Geometry: final body of the model. Coordinates: model frame, mm. A direction names the side the tool comes from. Give positions to 0.01 mm unless a question says otherwise; leave off trailing zeros. Write each loop counter-clockwise with the first axis right and the second up, starting at its lowest first coordinate (ties: lowest second). Pieces come first, ordered by that corner, then holes. Notation, with made-up numbers: (51, -19.75) -> (63, -19.75) arc R19 cw to (63, 7.25) -> close; hole circle Ø1 at (68, 58). An arc over 180 degrees is marked (long way). Answer as a JSON object with one key per item and string values. Group by question number.
(1) Material intervals for probe 1 along Z at (x, y) = (-48, -4) (3 decimals); probe 2 along X at (y, z) = (-2.4, -96.5); probe 3 along X at (y, z) = (-4.3, -36), sorted ascending.
(2) Section query A-A on x = -40.5. Output: boundary loops of the cut face in (y, z) (3 decimals), plus the area to 3 significant figures.
(3) Section query C-C on y = -1.8. State how many separate pieces and enclosed holes the cut face has, plus the area to 3 significant figures.
(4) Contact query for flat-ended pins moving along their axis: pin 1 Ø0.9 at (y, z) = (-3, 121) entering from +X; pin 2 Ø0.9 at (y, z) = (-2.5, -120.5) entering from -X; pin 3 Ø3 at (y, z) = (-3.5, 120.5) entering from -X; pin 4 Ø6 at (x, z) = (71.5, -25) entering from +Y. Output: stop coordinate, or through.
(5) Section query D-D on x = -102.5. Output: boundary loops of the cut face in (y, z), plus the area to 3 significant figures.
(6) Set-up query: faces 1 (the face through (108.388, -2.504, -63.727)), 2 (the face through (-125.48, -2.58, 27.77)). Return all of +Z, -Z, +X, -X, +Y, -Y with unobstructed straight access to the full face (end or side cutting, diameter ignored); none if empty.
(7) Section query B-B on z = 88. Output: boundary loops of the cut face in (x, y), plus the area to 3 significant figures.
(8) Draft query along X for faces 3 (the face through (125.21, -2.58, 28.24)), 4 (the face through (109.383, -2.504, 62.003)), 5 (the face through (-108.388, -2.504, 63.727)). Return one class per face: +X half, -X half, draft (parallel to the pull), parting line (faces both ways), or undercut.
from build123d import *

# Parameters (mm, degrees)
F1_DEPTH        = 5.08
F2_W            = 38.7485525078
F2_H            = 2.9464
F3_DEPTH        = 5.08
F3_COPIES_COUNT = 6


# Not quite as in the source:
# - a pattern or mirror of a feature is missing from the dataset's text; its kind, count and spacing are read off the source's solid


with BuildPart() as f1:
    # F0 (on Front) → F1 (new body)
    with BuildSketch(Plane.XZ):
        with BuildLine():
            Line((71.1237796615, 125.73), (-71.1237796615, 125.73))
            ThreePointArc((-71.1237796615, 125.73), (-72.3937796615, 125.3897045256), (-73.3234841871, 124.46))
            Line((-73.3234841871, 124.46), (-144.4472638486, 1.27))
            ThreePointArc((-144.4472638486, 1.27), (-144.7875593229, 0), (-144.4472638486, -1.27))
            Line((-144.4472638486, -1.27), (-73.3234841871, -124.46))
            ThreePointArc((-73.3234841871, -124.46), (-72.3937796615, -125.3897045256), (-71.1237796615, -125.73))
            Line((-71.1237796615, -125.73), (71.1237796615, -125.73))
            ThreePointArc((71.1237796615, -125.73), (72.3937796615, -125.3897045256), (73.3234841871, -124.46))
            Line((73.3234841871, -124.46), (144.4472638486, -1.27))
            ThreePointArc((144.4472638486, -1.27), (144.7875593229, 0), (144.4472638486, 1.27))
            Line((144.4472638486, 1.27), (73.3234841871, 124.46))
            ThreePointArc((73.3234841871, 124.46), (72.3937796615, 125.3897045256), (71.1237796615, 125.73))
        make_face()
    extrude(amount=F1_DEPTH)

    # F2 (on face) → F3 (cut, through all)
    with BuildSketch(Plane.XZ.offset(5.08)):
        with Locations((-38.4242762539, 121.0818)):
            Rectangle(F2_W, F2_H)
        with Locations((38.4242762539, 121.0818)):
            Rectangle(F2_W, F2_H)
    f3 = extrude(amount=-F3_DEPTH, mode=Mode.SUBTRACT)

    # F3_copies: F3 ×6 about axis
    f3_copies_axis = Axis((0, 0, 0), (0, 1, 0))
    for i in range(1, F3_COPIES_COUNT):
        add(f3.rotate(f3_copies_axis, i * 360 / F3_COPIES_COUNT), mode=Mode.SUBTRACT)


solid = f1.part
Answer list:
{
 "1": {"probe 1": "-125.73 to -122.555, -119.609 to 119.609, 122.555 to 125.73", "probe 2": "-89.47 to -85.8, -82.4 to 82.4, 85.8 to 89.47", "probe 3": "-124.4 to -120.73, -117.33 to 117.33, 120.73 to 124.4"},
 "2": {"outline": "(-5.08, -125.73) -> (0, -125.73) -> (0, -122.555) -> (-5.08, -122.555) -> close; (-5.08, -119.609) -> (0, -119.609) -> (0, 119.609) -> (-5.08, 119.609) -> close; (-5.08, 122.555) -> (0, 122.555) -> (0, 125.73) -> (-5.08, 125.73) -> close", "area": "1,250 mm2"},
 "3": {"separate pieces": "1", "enclosed holes": "12", "area": "53,400 mm2"},
 "4": {"pin 1": "x = 75.58", "pin 2": "x = -75.87", "pin 3": "x = -76.48", "pin 4": "y = 0"},
 "5": {"outline": "(-5.08, -73.92) -> (0, -73.92) -> (0, 73.92) -> (-5.08, 73.92) -> close", "area": "751 mm2"},
 "6": {"face 1": "-Z, +X, +Y, -Y", "face 2": "+Y, -Y"},
 "7": {"outline": "(-94.37, -5.08) -> (-90.71, -5.08) -> (-90.71, 0) -> (-94.37, 0) -> close; (-87.31, -5.08) -> (87.31, -5.08) -> (87.31, 0) -> (-87.31, 0) -> close; (90.71, -5.08) -> (94.37, -5.08) -> (94.37, 0) -> (90.71, 0) -> close", "area": "924 mm2"},
 "8": {"face 3": "undercut", "face 4": "+X half", "face 5": "-X half"}
}
